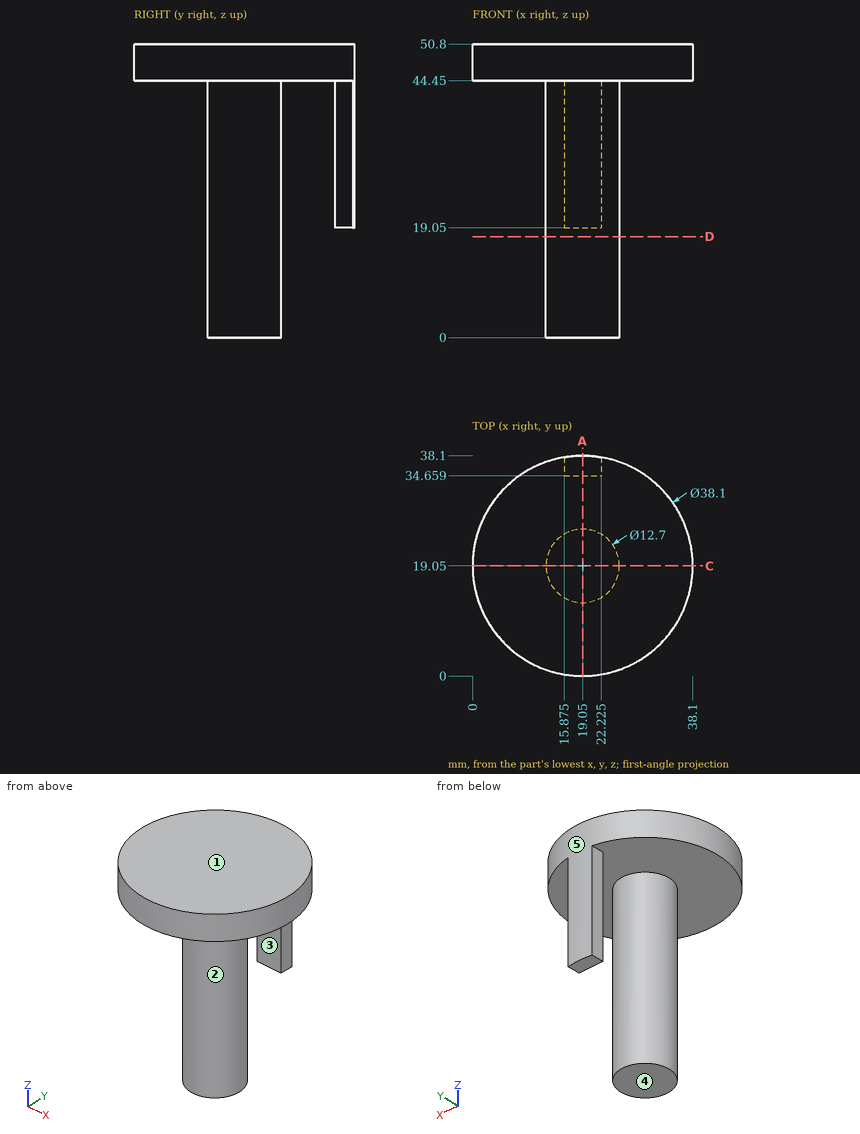
Answer from the drawing. Dimensions are ordinates in mm from the lowest x, y and z of the part. A direction names the side the tool comes from. Round coordinates to 2 decimals unless told otherwise and drop trailing zeros. Order: outer loops, then holes, each group sorted by start corner. A loop starts at its lowest first (then second) coordinate and runs counter-clockwise, first axis right, second up. Notation, with made-up numbers: (55.25, 29.5) - (96.25, 29.5) arc R22 ccw to (96.25, 50.5) - close; hole circle Ø11 at (76.5, 52.25). An arc over 180 degrees is marked (long way). Put each result on its own line as item: value. Start each with the question number.
(1) Find section A-A (x = 19.05). Give the vertices of the cut face in (y, z), plus the area to 3 significant figures.
(2) For the marked faces 1 and 2, determine the directions among +Z, -Z, +X, -X, +Y, -Y from which every point of the face is accessible in a straight line to the end or side of a thin tool.
(3) Determine the mould class of the marked faces 3, 4 and 5 for opening direction Y: released by +Y, released by -Y, zero draft, split by the parting line, or undercut.
(4) Straight lines are drawn through the part: probe 1 along Z at (x, y) = (33, 14); probe 2 along Y at (x, z) = (16, 23) (1 decimal); probe 3 along Y at (x, z) = (19, 13). For each, find the intervals that lie inside material, in ascending order. Write a range as from..to.
(5) Find section C-C (y = 19.05). Give the vertices of the cut face in (x, z).
(6) Find section D-D (z = 17.5). Give the vertices of the cut face in (x, y), plus the area to 3 significant figures.
(7) Given P1, Ø1.9, axis at x = 20.5, z = 34, coming from the -Y side; P2, Ø4, axis at x = 19, y = 35.5, coming from the -Z side; P3, Ø6, axis at y = 17.5, z = 7, coming from the +X side; P4, Ø8, axis at x = 23.5, y = 26, coming from the -Z side, each flat-ended and moving along its own axis, determine where each tip first touches the part or whether it passes through.
Reply:
1. outline: (0, 44.45) - (12.7, 44.45) - (12.7, 0) - (25.4, 0) - (25.4, 44.45) - (34.66, 44.45) - (34.66, 19.05) - (38.1, 19.05) - (38.1, 50.8) - (0, 50.8) - close
1. area: 894 mm^2
2. face 1: +Z, +X, -X, +Y, -Y
2. face 2: -Z
3. face 3: undercut
3. face 4: zero draft
3. face 5: split by the parting line
4. probe 1: 44.45..50.8
4. probe 2: 13.5..24.6, 34.7..37.9
4. probe 3: 12.7..25.4
5. outline: (0, 44.45) - (12.7, 44.45) - (12.7, 0) - (25.4, 0) - (25.4, 44.45) - (38.1, 44.45) - (38.1, 50.8) - (0, 50.8) - close
6. outline: circle Ø12.7 at (19.05, 19.05)
6. area: 127 mm^2
7. P1: y = 12.72
7. P2: z = 19.05
7. P3: x = 25.4
7. P4: z = 0
